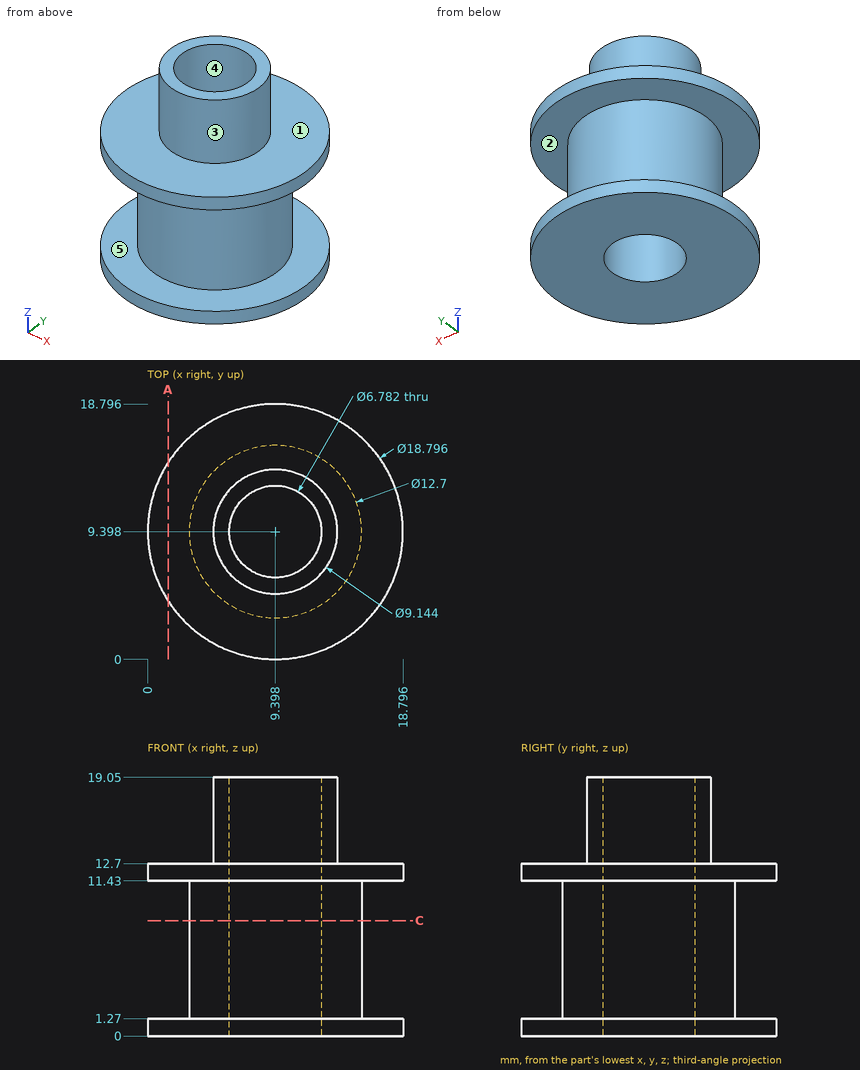
Could you check a few things on this drawing? It's one solid part, dimensions in mm from its lowest x, y, z. A direction names the side the tool comes from. Round coordinates to 2 decimals unless told otherwise and drop trailing zeros. Write each loop counter-clockwise with the first axis right and the second up, starting at its lowest first coordinate (ties: lowest second). Pieces come first, ordered by that corner, then holes. Notation, with made-up numbers: (3, -17.75) -> (58, -17.75) arc R27 cw to (58, 3.25) -> close; hole circle Ø10 at (16, 76.5). An arc over 180 degrees is marked (long way). One line per item, written item: value.
1) Suppose I cut it at A-A on x = 1.5. List the corners of the cut face in (y, z) for me.
Filled sheet:
outline: (4.3, 0) -> (14.49, 0) -> (14.49, 1.27) -> (4.3, 1.27) -> close; (4.3, 11.43) -> (14.49, 11.43) -> (14.49, 12.7) -> (4.3, 12.7) -> close
2) I'm going to push flat-ended pins straight in: pin 1 Ø8 at (x, z) = (5, 3.5) entering from +Y; pin 2 Ø5 at (y, z) = (16.5, 12.5) entering from +X; pin 3 Ø6 at (x, y) = (9.398, 9.398) entering from -Z; pin 4 Ø2 at (y, z) = (6.5, 11) entering from -X. Where does each tip first touch, or does it pass through?
Filled sheet:
pin 1: stops at y = 18.73
pin 2: stops at x = 17.59
pin 3: passes through
pin 4: stops at x = 0.21
3) We'd pull the mould along Z, two halves only. Please class the marked faces 1, 2 and 3: released by +Z, released by -Z, zero draft, split by the parting line, or undercut.
Filled sheet:
face 1: released by +Z
face 2: undercut
face 3: zero draft
4) For the marked faces 4 and 5, which set-ups out of +Z, -Z, +X, -X, +Y, -Y let a thin tool reach every point of the face, with its end or its side?
Filled sheet:
face 4: +Z, -Z
face 5: none
5) Suppose I cut it at C-C on z = 8.5. List the corners of the cut face in (x, y) for me.
Filled sheet:
outline: circle Ø12.7 at (9.4, 9.4); hole circle Ø6.78 at (9.4, 9.4)
6) If I drill on line 1 (Z direction, x = 10.5, y = 16.75); line 2 (Y direction, x = 9.5, z = 11.5); line 3 (X direction, y = 9.5, z = 8), over which ranges is the centre line in solid material (lowest first)? Write a range as [from, to].
Filled sheet:
line 1: z = [0, 1.27], [11.43, 12.7]
line 2: y = [0, 6.01], [12.79, 18.8]
line 3: x = [3.05, 6.01], [12.79, 15.75]
